Part model, mm, in its own coordinate system. A direction names the side the tool comes from. Round coordinates to 2 decimals unless told otherwise and drop trailing zeros. Order: outer loops, then holes, each group sorted by start corner. A loop starts at its lowest first (then second) coordinate and runs counter-clockwise, first axis right, second up. Notation, with made-up numbers: (69.25, 78.25) - (83.25, 78.25) arc R14 cw to (83.25, 90.25) - close; hole circle Ø3 at (20, 36.5). An arc over 180 degrees is marked (long way). Answer as a JSON object with one key per item and string values.
```python
from build123d import *

# Parameters (mm, degrees)
SKETCH1_W           = 12.7
SKETCH1_H           = 44.45
BOSS_EXTRUDE1_DEPTH = 3
FILLET1_R           = 3.175


with BuildPart() as part:
    # Sketch1 → Boss-Extrude1 (new, symmetric)
    with BuildSketch(Plane.XY):
        Rectangle(SKETCH1_W, SKETCH1_H)
        with BuildLine():
            Line((1.526908397, 15.875), (1.526908397, -15.875))
            ThreePointArc((1.526908397, -15.875), (0, -17.401908397), (-1.526908397, -15.875))
            Line((-1.526908397, -15.875), (-1.526908397, 15.875))
            ThreePointArc((-1.526908397, 15.875), (0, 17.401908397), (1.526908397, 15.875))
        make_face(mode=Mode.SUBTRACT)
    extrude(amount=BOSS_EXTRUDE1_DEPTH, both=True)

    # Fillet1
    fillet1_edges = [part.edges().sort_by_distance(p)[0] for p in [
        (6.35, -22.225, 0),
        (-6.35, -22.225, 0),
        (-6.35, 22.225, 0),
        (6.35, 22.225, 0),
    ]]
    fillet(fillet1_edges, radius=FILLET1_R)


solid = part.part
```
Item 1: Two-plate mould, pull along Y, no slides. Class faces 3 (the flat face through (3, 0, -3)), 4 (the flat face through (0, 22.225, 0)), 5 (the cylindrical face through (0, 17.4, 0)): pulls with the +Y half, pulls with the -Y half, needs draft (parallel to the pull), parting line crosses it, or undercut.
Taken from the geometry:
{"face 3": "needs draft", "face 4": "pulls with the +Y half", "face 5": "undercut"}
Item 2: Cut at C-C (x = 0). Write the cut outline in (y, z) (3 decimals).
Taken from the geometry:
{"outline": "(-22.225, -3) - (-17.402, -3) - (-17.402, 3) - (-22.225, 3) - close; (17.402, -3) - (22.225, -3) - (22.225, 3) - (17.402, 3) - close"}
Item 3: Cut at B-B (z = -1.6). Write the cut outline in (x, y) (3 decimals), plus the area to 3 significant figures.
Taken from the geometry:
{"outline": "(-6.35, -19.05) arc R3.175 ccw to (-3.175, -22.225) - (3.175, -22.225) arc R3.175 ccw to (6.35, -19.05) - (6.35, 19.05) arc R3.175 ccw to (3.175, 22.225) - (-3.175, 22.225) arc R3.175 ccw to (-6.35, 19.05) - close; hole (-1.527, -15.875) arc R1.527 ccw to (1.527, -15.875) - (1.527, 15.875) arc R1.527 ccw to (-1.527, 15.875) - close", "area": "452 mm2"}
Item 4: Tool access for faces 1 (the flat face through (-1.527, 0, 0)), 2 (the cylindrical face through (-5.445, -21.27, 0.042)): list every direction of +Z, -Z, +X, -X, +Y, -Y with a clear straight run to the whole face (end or side of a thin tool).
Taken from the geometry:
{"face 1": "+Z, -Z", "face 2": "+Z, -Z, -X, -Y"}
Item 5: Cut at A-A (y = 1). Write the cut outline in (x, z), plus the area to 3 significant figures.
Taken from the geometry:
{"outline": "(-6.35, -3) - (-1.53, -3) - (-1.53, 3) - (-6.35, 3) - close; (1.53, -3) - (6.35, -3) - (6.35, 3) - (1.53, 3) - close", "area": "57.9 mm2"}
Item 6: Probe L1, parallel to X at y = -12.5, z = -1.4; L2, parallel to Y at x = 3.25, z = 1.85; L3, parallel to Y at x = 4, z = 0.55. List the from-to ranges inside material, lowest first. Write a range as from..to.
Taken from the geometry:
{"L1": "-6.35..-1.53, 1.53..6.35", "L2": "-22.22..22.22", "L3": "-22.12..22.12"}
